Here's how the part is built. I have some questions about the finished solid (model axes, mm). A direction names the side the tool comes from. Give positions to 0.01 mm unless a question says otherwise; leave off trailing zeros. Write each loop counter-clockwise with the first axis right and the second up, starting at its lowest first coordinate (ties: lowest second). Pieces come first, ordered by that corner, then holes. Notation, with made-up numbers: (49.5, -19) -> (81.5, -19) arc R31 cw to (81.5, 13) -> close; hole circle Ø2 at (-30, -38). An arc over 180 degrees is marked (long way). Use one line per item in the form item = value.
Autodesk Inventor part; units mm, degrees
ref_plane "YZ Plane" through (0, 0, 0) normal (1, 0, 0) x (0, 1, 0)
ref_plane "XZ Plane" through (0, 0, 0) normal (0, 1, 0) x (-1, 0, 0)
ref_plane "XY Plane" through (0, 0, 0) normal (0, 0, 1) x (1, 0, 0)
sketch "スケッチ1" plane through (0, 0, 0) normal (0, 0, 1) x (1, 0, 0)
  line L0 (0, 0) -> (40, 0)
  line L1 (40, 0) -> (40, 40)
  line L2 (40, 40) -> (0, 40)
  line L3 (0, 40) -> (0, 0)
  dimension "d0" = 40
  dimension "d1" = 40
extrude "押し出し1" add sketch "スケッチ1" along normal blind 10
sketch "スケッチ2" plane through (0, 0, 10) normal (0, 0, 1) x (1, 0, 0)
  line L0 (40, 40) -> (0, 40)
  line L1 (40, 40) -> (25, 40)
  line L2 (25, 40) -> (25, 25)
  line L3 (25, 25) -> (40, 25)
  line L4 (40, 25) -> (40, 40)
  point P0 (0, 0)
  point P1 (25, 40)
  dimension "d4" = 15
  dimension "d5" = 15
extrude "押し出し2" cut sketch "スケッチ2" against normal blind 10
sketch "スケッチ3" plane through (0, 0, 10) normal (0, 0, 1) x (1, 0, 0)
  line L0 (0, 40) -> (15, 40)
  line L1 (15, 40) -> (15, 25)
  line L2 (15, 25) -> (0, 25)
  line L3 (0, 25) -> (0, 40)
  line L4 (0, 0) -> (40, 0)
  line L5 (0, 0) -> (15, 0)
  line L6 (15, 0) -> (15, 15)
  line L7 (15, 15) -> (0, 15)
  line L8 (0, 15) -> (0, 0)
  line L9 (40, 0) -> (25, 0)
  line L10 (25, 0) -> (25, 15)
  line L11 (25, 15) -> (40, 15)
  line L12 (40, 15) -> (40, 0)
  point P0 (25, 0)
  dimension "d8" = 15
  dimension "d9" = 15
  dimension "d10" = 15
  dimension "d11" = 15
  dimension "d12" = 15
  dimension "d13" = 15
extrude "押し出し3" cut sketch "スケッチ3" against normal blind 10
sketch "スケッチ4" plane through (25, 25, 10) normal (1, 0, 0) x (0, 0, -1)
  line L0 (0, 15) -> (10, 15)
  line L1 (10, 15) -> (10, 0)
  line L2 (10, -10) -> (10, -25)
  line L3 (10, -25) -> (0, -25)
  point P0 (5, 10)
  point P1 (5, -20)
  dimension "d16" = 5
  dimension "d17" = 5
  dimension "d18" = 5
  dimension "d19" = 5
hole "穴1" at (25, 35, 5) at (25, 5, 5) direction (-1, 0, 0) diameter 6 end through all
sketch "スケッチ5" plane through (0, 25, 10) normal (0, 1, 0) x (1, 0, 0)
  line L0 (0, 10) -> (15, 10)
  line L1 (0, 0) -> (0, 10)
  line L2 (25, 10) -> (40, 10)
  line L3 (40, 10) -> (40, 0)
  point P0 (5, 5)
  point P1 (35, 5)
  dimension "d27" = 5
  dimension "d28" = 5
  dimension "d29" = 5
  dimension "d30" = 5
hole "穴2" at (5, 25, 5) at (35, 25, 5) direction (0, -1, 0) diameter 6 end through all
sketch "スケッチ6" plane through (0, 0, 10) normal (0, 0, 1) x (1, 0, 0)
  line L0 (40, 15) -> (40, 25)
  line L1 (25, 40) -> (15, 40)
  point P0 (0, 0)
  point P1 (20, 20)
  dimension "d38" = 20
  dimension "d39" = 20
hole "穴3" at (20, 20, 10) direction (0, 0, -1) diameter 2.459 end through all
properties part number "シリンダ先端パーツ"
Q1. Which directions (+Z, -Z, +X, -X, +Y, -Y) give clear straight access to the entire face, cutting with the end or side of a thin tool? Please do faces 1 (the face through (9, 25, 5)), 2 (the face through (15, 9, 5)), 3 (the face through (25, 9, 5)), 4 (the face through (31, 25, 5)).
Result set:
face_1 = +Z, -Z, -X, +Y
face_2 = +Z, -Z, -X, -Y
face_3 = +Z, -Z, +X, -Y
face_4 = +Z, -Z, +X, +Y
Q2. I want a section at D-D, the plane z = 9. Write out the boundary of the cut face in (x, y).
Result set:
outline = (0, 15) -> (15, 15) -> (15, 0) -> (25, 0) -> (25, 15) -> (40, 15) -> (40, 25) -> (25, 25) -> (25, 40) -> (15, 40) -> (15, 25) -> (0, 25) -> close; hole circle Ø2.46 at (20, 20)
Q3. I want a section at B-B, the plane x = 20. Write out the boundary of the cut face in (y, z).
Result set:
outline = (0, 0) -> (18.77, 0) -> (18.77, 10) -> (0, 10) -> close; (21.23, 0) -> (40, 0) -> (40, 10) -> (21.23, 10) -> close; hole circle Ø6 at (5, 5); hole circle Ø6 at (35, 5)
Q4. If we mould it in two halves opening along Z, with no side actions, what happens to faces 5 (the face through (20, 16, 10)), 6 (the face through (2, 20, 5)), 7 (the face through (40, 20, 5))? For each: +Z half, -Z half, draft (parallel to the pull), parting line (faces both ways), or undercut.
Result set:
face_5 = +Z half
face_6 = undercut
face_7 = draft
Q5. If I drill on line 1 along Y through (x, z) = (24, 5); line 2 along Y through (x, z) = (20, 3.25), over which ranges is the centre line in solid material (lowest first)? Write a range as from..to.
Result set:
line_1 = 0..2, 8..32, 38..40
line_2 = 0..2.56, 7.44..18.77, 21.23..32.56, 37.44..40
Q6. I want a section at A-A, the plane z = 5. Count the separate pieces of the cut face and the enclosed holes in it, and give its area (3 significant figures).
Result set:
separate_pieces = 5
enclosed_holes = 1
area = 455 mm2
Q7. Will these pins go through, and if not, where does the flat tip stop? pin 1 Ø5 at (y, z) = (29.5, 4.5) entering from +X; pin 2 Ø5 at (y, z) = (30, 5) entering from -X; pin 3 Ø1 at (x, z) = (8, 7) entering from +Y; pin 4 Ø8 at (x, y) = (28.5, 12.5) entering from +Z.
Result set:
pin_1 = 25
pin_2 = 15
pin_3 = 25
pin_4 = 10
